```python
from build123d import *

# Parameters (mm, degrees)
F0_W     = 156
F0_H     = 196
F1_DEPTH = 22
F2_DEPTH = 4
F3_R     = 45
F4_DEPTH = 4


# Not quite as in the source:
# - ends of sketch curves that miss each other by under 0.0002 mm in the source are joined


with BuildPart() as f1:
    # F0 (on Top) → F1 (new body)
    with BuildSketch(Plane.XY):
        with Locations((0.9172109421, 20.8848945383)):
            Rectangle(F0_W, F0_H)
        with BuildLine():
            ThreePointArc((2.9672109421, 39.7739786876), (0.9172109421, 1.8848945383), (-1.1327890579, 39.7739786876))
            Line((-1.1327890579, 39.7739786876), (-1.1327890579, 41.8294366129))
            ThreePointArc((-1.1327890579, 41.8294366129), (0.914481977, 43.8848999875), (2.9672182077, 41.8348945383))
            Line((2.9672182077, 41.8348945383), (2.9672109421, 41.8294366129))
            Line((2.9672109421, 41.8294366129), (2.9672109421, 39.7739786876))
        make_face(mode=Mode.SUBTRACT)
    extrude(amount=F1_DEPTH)

    # F0 (on Top) → F2 (join)
    with BuildSketch(Plane.XY):
        with Locations((0.9172109421, 20.8848945383)):
            Rectangle(F0_W, F0_H)
        with BuildLine():
            ThreePointArc((2.9672109421, 39.7739786876), (0.9172109421, 1.8848945383), (-1.1327890579, 39.7739786876))
            Line((-1.1327890579, 39.7739786876), (-1.1327890579, 41.8294366129))
            ThreePointArc((-1.1327890579, 41.8294366129), (0.914481977, 43.8848999875), (2.9672182077, 41.8348945383))
            Line((2.9672182077, 41.8348945383), (2.9672109421, 41.8294366129))
            Line((2.9672109421, 41.8294366129), (2.9672109421, 39.7739786876))
        make_face(mode=Mode.SUBTRACT)
    extrude(amount=F2_DEPTH)

    # F3 (on face) → F4 (cut)
    with BuildSketch(Plane(origin=(0, 0, 0), x_dir=(1, 0, 0), z_dir=(0, 0, -1))):
        with Locations((0.9172109421, -20.8848945383)):
            Circle(F3_R)
    extrude(amount=-F4_DEPTH, mode=Mode.SUBTRACT)


solid = f1.part
```
Read the model definition and answer for the solid it produces. Units are mm, in the model's axes. A direction names the side the tool comes from. Give positions to 0.01 mm unless a question says otherwise; leave off trailing zeros. Write each loop counter-clockwise with the first axis right and the second up, starting at its lowest first coordinate (ties: lowest second). Pieces come first, ordered by that corner, then holes. Notation, with made-up numbers: M -36,8 L -14,8 A29 ccw -14,32 Z; hole C 45,62.5 d9. An arc over 180 degrees is marked long. Put each result on its own line as item: value. Start each with the question number.
1. Which of the six approach directions +Z, -Z, +X, -X, +Y, -Y give full straight-line access (tool end or side, diameter ignored) to faces 4 (the flat face through (20.3, 20.3, 4)), 5 (the flat face through (78.917, 20, 11)), 6 (the cylindrical face through (0.869, 43.884, 12.874))?
2. The part is cut by section B-B, the plane x = -4. Give the vertices of the cut face in (y, z).
3. For a pull along Y with two mould halves and no side action, classify faces 1 (the flat face through (0, -77.115, 11)), 2 (the cylindrical face through (1.7, 1.9, 12.9)), 3 (the flat face through (-18, 66, 0)) as released by +Y, released by -Y, zero draft, split by the parting line, or undercut.
4. This flat-tipped pin is pushed along its axis until it touches: pin 1 Ø3 at (x, y) = (15.5, 12.5) entering from -Z. Where does it stop, or does it pass through?
5. The part is cut by section D-D, the plane x = -31. Give the vertices of the cut face in (y, z), and give its area (3 significant figures).
6. Consider line 1 along Y through (x, z) = (0, 1.25); line 2 along Y through (x, z) = (12, 7); line 3 along X through (y, z) = (15, 6.5). Determine where each line is inside the solid, lowest interval first.
7. The part is cut by section C-C, the plane y = -9. Give the vertices of the cut face in (x, z).
Final values:
1. face 4: -Z
1. face 5: +Z, -Z, +X, +Y, -Y
1. face 6: +Z, -Z
2. outline: M -77.12,0 L -23.85,0 L -23.85,4 L 2.53,4 L 2.53,22 L -77.12,22 Z; M 39.24,4 L 65.62,4 L 65.62,0 L 118.88,0 L 118.88,22 L 39.24,22 Z
3. face 1: released by -Y
3. face 2: undercut
3. face 3: zero draft
4. pin 1: passes through
5. outline: M -77.12,0 L -10.84,0 L -10.84,4 L 52.61,4 L 52.61,0 L 118.88,0 L 118.88,22 L -77.12,22 Z
5. area: 4,060 mm²
6. line 1: y = -77.12 to -24.11, 65.88 to 118.88
6. line 2: y = -77.12 to 5.45, 36.32 to 118.88
6. line 3: x = -77.08 to -17.15, 18.98 to 78.92
7. outline: M -77.08,0 L -32.73,0 L -32.73,4 L 34.56,4 L 34.56,0 L 78.92,0 L 78.92,22 L -77.08,22 Z
